from build123d import *

# Parameters (mm, degrees)
SKETCH1_W                      = 127
SKETCH1_H                      = 247
BOSS_EXTRUDE1_DEPTH            = 63.5
M3X0_5_TAPPED_HOLE1_AT_2_COUNT = 2
M3X0_5_TAPPED_HOLE1_AT_2_PITCH = 220.907220344
M3X0_5_TAPPED_HOLE1_AT_3_COUNT = 2
M3X0_5_TAPPED_HOLE1_AT_3_PITCH = 20
M3X0_5_TAPPED_HOLE1_AT_4_COUNT = 2
M3X0_5_TAPPED_HOLE1_AT_4_PITCH = 220
SKETCH5_W                      = 33.332781188
SKETCH5_H                      = 14.481960758
BOSS_EXTRUDE2_DEPTH            = 15
SKETCH6_W                      = 81.228427944
SKETCH6_H                      = 10.113101088
BOSS_EXTRUDE3_DEPTH            = 17


with BuildPart() as part:
    # Sketch1 → Boss-Extrude1 (new body)
    with BuildSketch(Plane(origin=(0, 0, 0), x_dir=(1, 0, 0), z_dir=(0, 1, 0))):
        Rectangle(SKETCH1_W, SKETCH1_H)
    extrude(amount=BOSS_EXTRUDE1_DEPTH)

    # Sketch4 → M3x0.5 Tapped Hole1 (revolve, cut)
    with BuildSketch(Plane(origin=(63.5, 50, 112.5), x_dir=(0, 0, -1), z_dir=(0, 1, 0))):
        Polygon((0, 0), (0, 4.751075774), (1.25, 4), (1.25, 0), align=None)
    m3x0_5_tapped_hole1 = revolve(axis=Axis((69.85, 50, 112.5), (-1, 0, 0)), mode=Mode.SUBTRACT)

    # M3x0.5 Tapped Hole1 at 2: M3x0.5 Tapped Hole1 ×2
    with Locations(*[Vector(0, -0.09053574604251853, -0.9958932064677039) * (i * M3X0_5_TAPPED_HOLE1_AT_2_PITCH) for i in range(1, M3X0_5_TAPPED_HOLE1_AT_2_COUNT)]):
        add(m3x0_5_tapped_hole1, mode=Mode.SUBTRACT)

    # M3x0.5 Tapped Hole1 at 3: M3x0.5 Tapped Hole1 ×2
    with Locations(*[(0, -i * M3X0_5_TAPPED_HOLE1_AT_3_PITCH, 0) for i in range(1, M3X0_5_TAPPED_HOLE1_AT_3_COUNT)]):
        add(m3x0_5_tapped_hole1, mode=Mode.SUBTRACT)

    # M3x0.5 Tapped Hole1 at 4: M3x0.5 Tapped Hole1 ×2
    with Locations(*[(0, 0, -i * M3X0_5_TAPPED_HOLE1_AT_4_PITCH) for i in range(1, M3X0_5_TAPPED_HOLE1_AT_4_COUNT)]):
        add(m3x0_5_tapped_hole1, mode=Mode.SUBTRACT)

    # Sketch5 → Boss-Extrude2 (add)
    with BuildSketch(Plane.XY.offset(123.5)):
        with Locations((-29.125731135, 44.621088627)):
            Rectangle(SKETCH5_W, SKETCH5_H)
    extrude(amount=BOSS_EXTRUDE2_DEPTH)

    # Sketch6 → Boss-Extrude3 (add)
    with BuildSketch(Plane(origin=(0, 0, -123.5), x_dir=(-1, 0, 0), z_dir=(0, 0, -1))):
        with Locations((0.809048087, 44.806195806)):
            Rectangle(SKETCH6_W, SKETCH6_H)
    extrude(amount=BOSS_EXTRUDE3_DEPTH)

    # Mirror1: M3x0.5 Tapped Hole1 across plane
    add(m3x0_5_tapped_hole1.mirror(Plane(origin=(0, 0, 0), x_dir=(0, 0, 1), z_dir=(1, 0, 0))), mode=Mode.SUBTRACT)

    # Mirror1 copy 1 sketch → Mirror1 copy 1 (revolve, cut)
    with BuildSketch(Plane(origin=(-63.5, 30, -107.5), x_dir=(0, 0, -1), z_dir=(0, 1, 0))):
        Polygon((0, 0), (0, -4.751075774), (1.25, -4), (1.25, 0), align=None)
    revolve(axis=Axis((-69.85, 30, -107.5), (-1, 0, 0)), mode=Mode.SUBTRACT)

    # Mirror1 copy 2 sketch → Mirror1 copy 2 (revolve, cut)
    with BuildSketch(Plane(origin=(-63.5, 30, 112.5), x_dir=(0, 0, -1), z_dir=(0, 1, 0))):
        Polygon((0, 0), (0, -4.751075774), (1.25, -4), (1.25, 0), align=None)
    revolve(axis=Axis((-69.85, 30, 112.5), (-1, 0, 0)), mode=Mode.SUBTRACT)

    # Mirror1 copy 3 sketch → Mirror1 copy 3 (revolve, cut)
    with BuildSketch(Plane(origin=(-63.5, 50, -107.5), x_dir=(0, 0, -1), z_dir=(0, 1, 0))):
        Polygon((0, 0), (0, -4.751075774), (1.25, -4), (1.25, 0), align=None)
    revolve(axis=Axis((-69.85, 50, -107.5), (-1, 0, 0)), mode=Mode.SUBTRACT)


solid = part.part
Build history of the part. All positions in model axes, mm. A direction names the side the tool comes from. Coordinates: 2 decimals unless noted, no trailing zeros. Order: outer loops, then holes, each group sorted by start corner. A loop starts at its lowest first (then second) coordinate and runs counter-clockwise, first axis right, second up. Notation, with made-up numbers: (-18.75, 80) - (6.25, 80) arc R23 ccw to (6.25, 116) - close; hole circle Ø3 at (3, 47.5). An arc over 180 degrees is marked (long way). Put each result on its own line as item: value.
1. Tool access for faces 1 (the face through (-45.792, 45, 131)), 2 (the face through (-29, 51.862, 131)), 3 (the face through (-29, 37.38, 131)), 4 (the face through (-41.423, 45, -132)): list every direction of +Z, -Z, +X, -X, +Y, -Y with a clear straight run to the whole face (end or side of a thin tool).
Answer sheet:
face 1: +Z, -X, +Y, -Y
face 2: +Z, +X, -X, +Y
face 3: +Z, +X, -X, -Y
face 4: -Z, -X, +Y, -Y
2. Saw through at C-C (x = 43.5). Write the cut outline in (y, z), and give its area (3 significant figures).
Answer sheet:
outline: (0, -123.5) - (63.5, -123.5) - (63.5, 123.5) - (0, 123.5) - close
area: 15,700 mm^2
3. Probe line 1 along Z through (x, y) = (61, 50); line 2 along Y through (x, z) = (-61.2, 112.5); line 3 along Z through (x, y) = (-4, 24.5). List the from-to ranges inside material, lowest first. Write a range as [from, to].
Answer sheet:
line 1: z = [-123.5, -108.75], [-106.25, 111.25], [113.75, 123.5]
line 2: y = [0, 28.75], [31.25, 48.75], [51.25, 63.5]
line 3: z = [-123.5, 123.5]
4. Saw through at B-B (y = 16). Write the cut outline in (x, z).
Answer sheet:
outline: (-63.5, -123.5) - (63.5, -123.5) - (63.5, 123.5) - (-63.5, 123.5) - close
5. Drop flat-ended pins along their axis: P1, Ø11, axis at y = 44.5, z = -131.5, coming from the +X side; P2, Ø18.5, axis at x = -18.5, z = -135, coming from the +Y side; P3, Ø6, axis at x = -8, y = 25.5, coming from the +Z side. Give the stop position or say it passes through.
Answer sheet:
P1: stops at x = 39.81
P2: stops at y = 49.86
P3: stops at z = 123.5
6. Saw through at A-A (x = 10). Write the cut outline in (y, z), and give its area (3 significant figures).
Answer sheet:
outline: (0, -123.5) - (39.75, -123.5) - (39.75, -140.5) - (49.86, -140.5) - (49.86, -123.5) - (63.5, -123.5) - (63.5, 123.5) - (0, 123.5) - close
area: 15,900 mm^2
